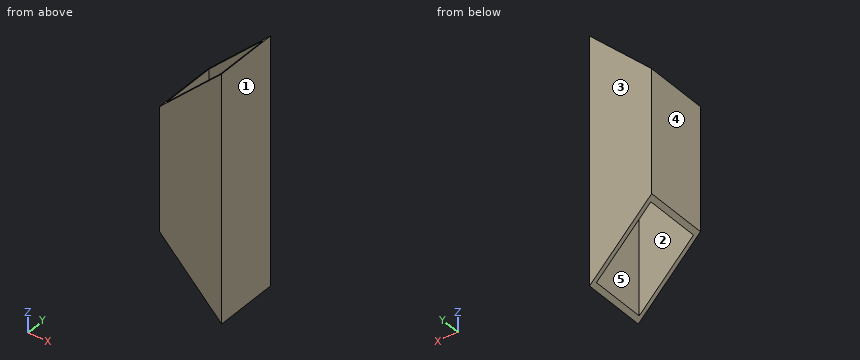
Autodesk Inventor part; units mm, degrees
ref_plane "YZ Plane" through (0, 0, 0) normal (1, 0, 0) x (0, 1, 0)
ref_plane "XZ Plane" through (0, 0, 0) normal (0, 1, 0) x (-1, 0, 0)
ref_plane "XY Plane" through (0, 0, 0) normal (0, 0, 1) x (1, 0, 0)
sketch "Sketch1" plane through (0, 0, 0) normal (0, 0, 1) x (1, 0, 0)
  line L0 (0, 0) -> (25.4, 0)
  line L1 (25.4, 0) -> (25.4, 25.4)
  line L2 (25.4, 25.4) -> (0, 25.4)
  line L3 (0, 25.4) -> (0, 0)
  dimension "d0" = 25.4
  dimension "d1" = 25.4
extrude "Extrusion1" add sketch "Sketch1" along normal blind 101.6
shell "Shell1" thickness 1.5875 removed faces 2 at (8.4667, 16.9333, 0) at (8.4667, 16.9333, 101.6)
sketch "Sketch2" plane through (0, 25.4, 0) normal (0, 1, 0) x (1, 0, 0)
  line L0 (0, -101.6) -> (25.4, -101.6)
  line L1 (25.4, 0) -> (0, 0)
  line L2 (0, 0) -> (0, -101.6)
  line L3 (25.4, 0) -> (0, -25.4)
  line L4 (0, -25.4) -> (0, 0)
  line L5 (0, 0) -> (25.4, 0)
  line L6 (25.4, -101.6) -> (0, -76.2)
  line L7 (0, -101.6) -> (0, -76.2)
  line L8 (0, -101.6) -> (25.4, -101.6)
  dimension "d5" = 45
  dimension "d6" = 45
extrude "Extrusion2" cut sketch "Sketch2" against normal through all
properties part number "Frame_VerticalAngle_Mid" material "Aluminum-6061"
Input: part model. Units: mm. Frame: model coordinates. Face numbers are marked on the shaded views. A direction names the side the tool comes from. Give positions to 0.01 mm unless a question says otherwise; leave off trailing zeros. Order: outer loops, then holes, each group sorted by start corner. A loop starts at its lowest first (then second) coordinate and runs counter-clockwise, first axis right, second up. Notation, with made-up numbers: (6, 33) -> (37, 33) arc R21 cw to (37, 66) -> close; hole circle Ø5 at (-27.5, 85.5). An arc over 180 degrees is marked (long way). Use one line per item in the form item = value.
1) Section C-C, the plane z = 11. Return loops of the section in (x, y).
Response values:
outline = (14.4, 0) -> (25.4, 0) -> (25.4, 25.4) -> (14.4, 25.4) -> (14.4, 23.81) -> (23.81, 23.81) -> (23.81, 1.59) -> (14.4, 1.59) -> close
2) Line query: probe 1 along X at (y, z) = (8, 56); probe 2 along X at (y, z) = (5, 12). Output: solid intervals per line, ascending.
Response values:
probe_1 = 0 to 1.59, 23.81 to 25.4
probe_2 = 23.81 to 25.4
3) Section B-B, the plane y = 21.75. Return loops of the section in (x, z).
Response values:
outline = (0, 25.4) -> (1.59, 23.81) -> (1.59, 77.79) -> (0, 76.2) -> close; (23.81, 1.59) -> (25.4, 0) -> (25.4, 101.6) -> (23.81, 100.01) -> close
4) Mould query, pull axis X, two halves, no side actions, for the marked faces 1, 2 and 3. Classes: pulls with the +X half, pulls with the -X half, needs draft (parallel to the pull), parting line crosses it, or undercut.
Response values:
face_1 = pulls with the +X half
face_2 = undercut
face_3 = needs draft
5) Section A-A, the plane x = 4.75. Return loops of the section in (y, z), and give its area (3 significant figures).
Response values:
outline = (0, 20.65) -> (1.59, 20.65) -> (1.59, 80.95) -> (0, 80.95) -> close; (23.81, 20.65) -> (25.4, 20.65) -> (25.4, 80.95) -> (23.81, 80.95) -> close
area = 191 mm^2
6) Reachability of the marked faces 4 and 5 from +Z, -Z, +X, -X, +Y, -Y: full face, straight path, thin tool, end or side. Return the list, or none.
Response values:
face_4 = +Z, -Z, -X, +Y, -Y
face_5 = +Z, -Z
7) First-contact query: pin 1 Ø3 at (x, y) = (3, 14.5) entering from +Z; pin 2 Ø12 at (x, y) = (6, 15.5) entering from -Z. Flat tips, straight axial feed; report the tip coordinate or a pass-through.
Response values:
pin_1 = 77.79
pin_2 = 23.81
8) Section D-D, the plane z = 63. Return loops of the section in (x, y).
Response values:
outline = (0, 0) -> (25.4, 0) -> (25.4, 25.4) -> (0, 25.4) -> close; hole (1.59, 1.59) -> (23.81, 1.59) -> (23.81, 23.81) -> (1.59, 23.81) -> close
